For this review, take the finished solid that the model builds, in its own axes (mm). Coordinates: 2 decimals unless noted, no trailing zeros. Write each loop counter-clockwise with the first axis right and the second up, starting at its lowest first coordinate (ties: lowest second). Pieces come first, ordered by that corner, then holes. Notation, with made-up numbers: (-36.75, 80) -> (-24.75, 80) arc R26 ccw to (-24.75, 115) -> close; hole circle Ø1 at (59, 72.5). An arc over 180 degrees is marked (long way). Put each result on its own line as item: value. Start each with the question number.
Item 1: The part is to be moulded in two halves that separate along X. For faces 1 (the cylindrical face through (2, 3, 1554)), 2 (the cylindrical face through (2, 3, 1548)), 3 (the flat face through (-2, -245, 1550)), say which applies: +X half, -X half, draft (parallel to the pull), parting line (faces both ways), or undercut.
Item 2: Consider section B-B on x = 83.5. Give the boundary of the cut face in (y, z), and give its area (3 significant figures).
Item 3: To check wall thickness, follow L1, parallel to Z at x = -63.5, y = -21; L2, parallel to Z at x = 50.5, y = -128. State the ranges of each line that lie inside material, in increasing order.
Item 4: Insertion check: P1, Ø5, axis at x = -101.5, y = 123, coming from the -Z side; P2, Ø3.5, axis at x = -150.92, y = 220, coming from the -Z side; P3, Ø4, axis at y = 116, z = 1545, coming from the -X side. Each pin has a flat end and moves straight along its axis. Give the tip position at first contact, or say it passes through.
Item 5: Consider section A-A on y = 197. Give the boundary of the cut face in (x, z).
```python
from build123d import *

# Parameters (mm, degrees)
F0_W     = 490
F0_H     = 6
F1_ANGLE = 13
F4_D     = 6
F4_DEPTH = 100


with BuildPart() as f1:
    # F0 (on Right) → F1 (revolve, symmetric)
    with BuildSketch(Plane.YZ) as f1_sk:
        with Locations((0, 1551)):
            Rectangle(F0_W, F0_H)
    revolve(axis=Axis((0, -0.207613, 0), (0, 1, 0)), revolution_arc=F1_ANGLE / 2)
    revolve(f1_sk.sketch, axis=Axis((0, -0.207613, 0), (0, -1, 0)), revolution_arc=F1_ANGLE / 2)

    # F4
    with Locations(Plane.XY.offset(1600)):
        with Locations((-150.917794, 220), (150.917794, -220)):
            Hole(F4_D / 2, depth=F4_DEPTH)


solid = f1.part
```
Return value:
1. face 1: parting line
1. face 2: undercut
1. face 3: draft
2. outline: (-245, 1545.75) -> (245, 1545.75) -> (245, 1551.76) -> (-245, 1551.76) -> close
2. area: 2,940 mm^2
3. L1: 1546.7 to 1552.7
3. L2: 1547.18 to 1553.18
4. P1: z = 1544.5
4. P2: through
4. P3: x = -175.92
5. outline: (-175.92, 1544.01) -> (-175.24, 1538.05) arc R1548 cw to (175.24, 1538.05) -> (175.92, 1544.01) arc R1554 ccw to start
